Input: part model. Units: mm. Frame: model coordinates. Round coordinates to 2 decimals unless told otherwise and drop trailing zeros. Loops run counter-clockwise (first coordinate to the right, second up) from the corner with the lowest first, then second, coordinate; pieces in that order, holes last. Notation, with made-up numbers: (24, 64) -> (33, 64) arc R28 cw to (33, 97) -> close; hole circle Ø3 at (63, 8.25). An arc over 180 degrees is marked (long way). Answer as a JSON object with one key per item and string values. Group by question number.
Item 1: Section query A-A on x = 0. Return loops of the section in (y, z), and give its area (3 significant figures).
Item 2: Section query C-C on z = -390.5. Return loops of the section in (x, y), and give its area (3 significant figures).
Item 3: Pin query (flat end, axial travel): pin 1 (1 mm diameter, centred on x = -9, z = -461.5, fed in from +Y); pin 2 (2 mm diameter, centred on y = -5.5, z = -284.5, fed in from -X); pin 3 (1 mm diameter, centred on x = 4.5, z = -341, fed in from +Y). Return the tip coordinate at first contact, or that it passes through.
Item 4: Material intervals for line 1 (Z direction, x = -7.5, y = 7); line 2 (Y direction, x = -1.75, z = -716); line 3 (X direction, y = 1.25, z = 28), sorted ascending. Write a range as [from, to].
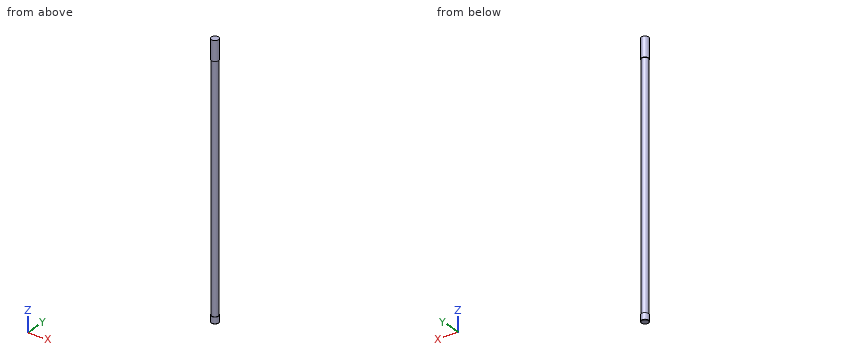
from build123d import *

# Parameters (mm, degrees)
ESQUISSE1_R        = 11.4
BOSS_EXTRU_1_DEPTH = 60
ESQUISSE2_R        = 10
BOSS_EXTRU_2_DEPTH = 750
ESQUISSE3_R        = 11.4
BOSS_EXTRU_3_DEPTH = 20
CONG_1_R           = 1


with BuildPart() as part:
    # Esquisse1 → Boss.-Extru.1 (new body)
    with BuildSketch(Plane.XY):
        Circle(ESQUISSE1_R)
    extrude(amount=BOSS_EXTRU_1_DEPTH)

    # Esquisse2 → Boss.-Extru.2 (add)
    with BuildSketch(Plane(origin=(0, 0, 0), x_dir=(-1, 0, 0), z_dir=(0, 0, -1))):
        Circle(ESQUISSE2_R)
    extrude(amount=BOSS_EXTRU_2_DEPTH)

    # Esquisse3 → Boss.-Extru.3 (add)
    with BuildSketch(Plane(origin=(0, 0, -750), x_dir=(-1, 0, 0), z_dir=(0, 0, -1))):
        with Locations(Location((0, 0, 0), (0, 0, 180))):
            Circle(ESQUISSE3_R)
    extrude(amount=-BOSS_EXTRU_3_DEPTH)

    # Congé1
    cong_1_edges = [part.edges().sort_by_distance(p)[0] for p in [
        (-11.4, 0, -750),
    ]]
    fillet(cong_1_edges, radius=CONG_1_R)


solid = part.part
Solved:
{
 "1": {"outline": "(-11.4, -749) arc R1 ccw to (-10.4, -750) -> (10.4, -750) arc R1 ccw to (11.4, -749) -> (11.4, -730) -> (10, -730) -> (10, 0) -> (11.4, 0) -> (11.4, 60) -> (-11.4, 60) -> (-11.4, 0) -> (-10, 0) -> (-10, -730) -> (-11.4, -730) -> close", "area": "16,400 mm²"},
 "2": {"outline": "circle Ø20 at (0, 0)", "area": "314 mm²"},
 "3": {"pin 1": "y = 5.27", "pin 2": "x = -8.93", "pin 3": "y = 9.17"},
 "4": {"line 1": "[-750, -730], [0, 60]", "line 2": "[-9.85, 9.85]", "line 3": "[-11.33, 11.33]"}
}
